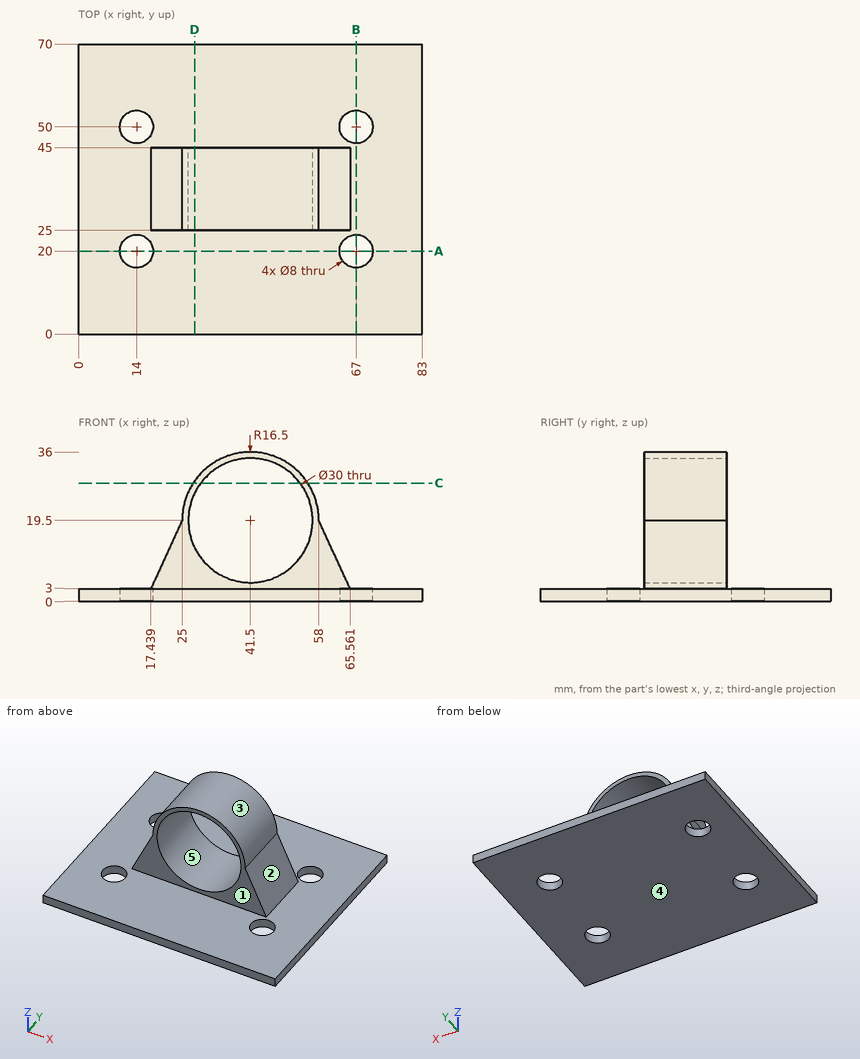
Study the drawing (mm; zero at the part's minimum x, y, z) and answer. A direction names the side the tool comes from. Round coordinates to 2 decimals unless told otherwise and drop trailing zeros. Write each loop counter-clockwise with the first axis right and the second up, starting at its lowest first coordinate (ties: lowest second). Pieces come first, ordered by that corner, then holes.
Q1. Find section B-B on x = 67. Determine the outline of the cut face in (y, z).
Values:
outline: (0, 0) - (16, 0) - (16, 3) - (0, 3) - close; (24, 0) - (46, 0) - (46, 3) - (24, 3) - close; (54, 0) - (70, 0) - (70, 3) - (54, 3) - close
Q2. The mould has two halves that part along X. Classify the marked faces 3, 4 and 5: released by +X, released by -X, zero draft, split by the parting line, or undercut.
Values:
face 3: split by the parting line
face 4: zero draft
face 5: undercut
Q3. Find section D-D on x = 28. Determine the outline of the cut face in (y, z).
Values:
outline: (0, 0) - (70, 0) - (70, 3) - (45, 3) - (45, 12.96) - (25, 12.96) - (25, 3) - (0, 3) - close; (25, 26.04) - (45, 26.04) - (45, 28.99) - (25, 28.99) - close
Q4. Find section A-A on y = 20. Determine the outline of the cut face in (x, z).
Values:
outline: (0, 0) - (10, 0) - (10, 3) - (0, 3) - close; (18, 0) - (63, 0) - (63, 3) - (18, 3) - close; (71, 0) - (83, 0) - (83, 3) - (71, 3) - close
Q5. Straight lines are drawn through the part: line 1 (Y direction, x = 14, z = 0.7); line 2 (X direction, y = 50, z = 1.4); line 3 (Z direction, x = 41, y = 32). For each, find the intervals that lie inside material, in ascending order.
Values:
line 1: y = 0 to 16, 24 to 46, 54 to 70
line 2: x = 0 to 10, 18 to 63, 71 to 83
line 3: z = 0 to 4.51, 34.49 to 35.99
Q6. A tool of negligible diameter and unlimited length cuts with its end or side. For the marked faces 1 and 2, from which of +Z, -Z, +X, -X, +Y, -Y can it reach the whole face along a straight path? Write none if from no direction.
Values:
face 1: +Z, +X, -X, -Y
face 2: +Z, +X, +Y, -Y
Q7. Find section C-C on z = 28.5. Determine the outline of the cut face in (x, y).
Values:
outline: (27.67, 25) - (29.5, 25) - (29.5, 45) - (27.67, 45) - close; (53.5, 25) - (55.33, 25) - (55.33, 45) - (53.5, 45) - close
Q8. Flat-ended cylindrical pins translate along their axes: P1, Ø2, axis at x = 35.5, y = 15.5, coming from the +Z side; P2, Ø4, axis at x = 29, y = 45.5, coming from the +Z side (1 decimal); P3, Ø2, axis at x = 54.5, y = 31.5, coming from the +Z side (1 decimal). Find the tip coordinate at first contact, or state that the pin passes through.
Values:
P1: stops at z = 3
P2: stops at z = 32.2
P3: stops at z = 30.8
